Build history of the part. All positions in model axes, mm. Round coordinates to 2 decimals unless told otherwise and drop trailing zeros. Write each loop counter-clockwise with the first axis right and the second up, starting at its lowest first coordinate (ties: lowest second). Pieces come first, ordered by that corner, then holes. Notation, with made-up numbers: (14, -5) - (47, -5) arc R22 ccw to (47, 22) - close; hole circle Ø1 at (40.25, 68). An arc over 180 degrees is marked (long way). Answer as a JSON object with one key per item and string values. Group by question number.
Item 1: Slice it at D-D, the plane z = 3.25. List the corners of the cut face in (x, y).
Item 2: Slice it at C-C, the plane y = 1.6. List the corners of the cut face in (x, z) (3 decimals).
Item 3: Two-plate mould, pull along Z, no slides. Class faces 1 (the flat face through (0, 2.5, 0)), 2 (the flat face through (0, 0, 9.835)), 3 (the cylindrical face through (21.8, 0, -2.4)), 4 (the cylindrical face through (-28.2, 0, -2.4)): +Z half, -Z half, draft (parallel to the pull), parting line (faces both ways), or undercut.
Item 4: Probe line 1 (X direction, y = -1.15, z = -0.25); line 2 (Z direction, x = -25, y = 0.3) (3 decimals); line 3 (X direction, y = 2.1, z = -2.5). List the from-to ranges inside material, lowest first. Write a range as from..to.
Item 5: Slice it at B-B, the plane x = -26.5. List the corners of the cut face in (y, z).
Item 6: Slice it at A-A, the plane z = 0. List the corners of the cut face in (x, y) (3 decimals).
Item 7: Flat gauge pins, fed straight in: pin 1 (2 mm diameter, centred on y = 0.5, z = 3.5, fed in from -X); pin 2 (3 mm diameter, centred on y = 0.5, z = -6, fed in from +X); pin 3 (2 mm diameter, centred on y = -0.5, z = -3.5, fed in from +X). Where does each tip first touch, or does it go through?
from build123d import *

# Parameters (mm, degrees)
F0_R     = 4
F1_DEPTH = 2.5


with BuildPart() as f1:
    # F0 (on Front) → F1 (new body, symmetric)
    with BuildSketch(Plane.XZ):
        with BuildLine():
            Line((0, 9.835), (-25, 9.835))
            ThreePointArc((-25, 9.835), (-34.835, 0), (-25, -9.835))
            Line((-25, -9.835), (0, -9.835))
            Line((0, -9.835), (25, -9.835))
            ThreePointArc((25, -9.835), (34.835, 0), (25, 9.835))
            Line((25, 9.835), (0, 9.835))
        make_face()
        with Locations((-25, 0)):
            Circle(F0_R, mode=Mode.SUBTRACT)
        with Locations((25, 0)):
            Circle(F0_R, mode=Mode.SUBTRACT)
    extrude(amount=F1_DEPTH, both=True)


solid = f1.part
Geometry says:
{
 "1": {"outline": "(-34.28, -2.5) - (-27.33, -2.5) - (-27.33, 2.5) - (-34.28, 2.5) - close; (-22.67, -2.5) - (22.67, -2.5) - (22.67, 2.5) - (-22.67, 2.5) - close; (27.33, -2.5) - (34.28, -2.5) - (34.28, 2.5) - (27.33, 2.5) - close"},
 "2": {"outline": "(-25, -9.835) - (25, -9.835) arc R9.835 ccw to (25, 9.835) - (-25, 9.835) arc R9.835 ccw to start; hole circle Ø8 at (-25, 0); hole circle Ø8 at (25, 0)"},
 "3": {"face 1": "draft", "face 2": "+Z half", "face 3": "undercut", "face 4": "undercut"},
 "4": {"line 1": "x = -34.83..-28.99, -21.01..21.01, 28.99..34.83", "line 2": "z = -9.835..-4, 4..9.835", "line 3": "x = -34.51..-28.12, -21.88..21.88, 28.12..34.51"},
 "5": {"outline": "(-2.5, -9.72) - (2.5, -9.72) - (2.5, -3.71) - (-2.5, -3.71) - close; (-2.5, 3.71) - (2.5, 3.71) - (2.5, 9.72) - (-2.5, 9.72) - close"},
 "6": {"outline": "(-34.835, -2.5) - (-29, -2.5) - (-29, 2.5) - (-34.835, 2.5) - close; (-21, -2.5) - (21, -2.5) - (21, 2.5) - (-21, 2.5) - close; (29, -2.5) - (34.835, -2.5) - (34.835, 2.5) - (29, 2.5) - close"},
 "7": {"pin 1": "stops at x = -34.51", "pin 2": "stops at x = 33.75", "pin 3": "stops at x = 34.51"}
}
